from build123d import *

# Parameters (mm, degrees)
SKETCH_1_W      = 3
SKETCH_1_H      = 8
SKETCH_1_W_2    = 8
SKETCH_1_H_2    = 3
EXTRUDE_1_DEPTH = 5


with BuildPart() as part:
    # Эскиз1 → Бобышка-Вытянуть1 (new body)
    with BuildSketch(Plane.XY):
        with BuildLine():
            Line((-31.75, 40.340066927), (-42.5, 40.340066927))
            ThreePointArc((-42.5, 40.340066927), (-43.914213562, 39.754280489), (-44.5, 38.340066927))
            Line((-44.5, 38.340066927), (-44.5, 27.590066927))
            Line((-44.5, 27.590066927), (-42, 27.590066927))
            Line((-42, 27.590066927), (-42, 30.090066927))
            Line((-42, 30.090066927), (-39.5, 30.090066927))
            Line((-39.5, 30.090066927), (-39.5, 21.590066927))
            Line((-39.5, 21.590066927), (-42, 21.590066927))
            Line((-42, 21.590066927), (-42, 24.090066927))
            Line((-42, 24.090066927), (-44.5, 24.090066927))
            Line((-44.5, 24.090066927), (-44.5, -32.409933073))
            Line((-44.5, -32.409933073), (-42, -32.409933073))
            Line((-42, -32.409933073), (-42, -29.909933073))
            Line((-42, -29.909933073), (-39.5, -29.909933073))
            Line((-39.5, -29.909933073), (-39.5, -38.409933073))
            Line((-39.5, -38.409933073), (-42, -38.409933073))
            Line((-42, -38.409933073), (-42, -35.909933073))
            Line((-42, -35.909933073), (-44.5, -35.909933073))
            Line((-44.5, -35.909933073), (-44.5, -46.659933073))
            ThreePointArc((-44.5, -46.659933073), (-43.914213562, -48.074146635), (-42.5, -48.659933073))
            Line((-42.5, -48.659933073), (-31.75, -48.659933073))
            Line((-31.75, -48.659933073), (-31.75, -46.159933073))
            Line((-31.75, -46.159933073), (-34.25, -46.159933073))
            Line((-34.25, -46.159933073), (-34.25, -43.659933073))
            Line((-34.25, -43.659933073), (-25.75, -43.659933073))
            Line((-25.75, -43.659933073), (-25.75, -46.159933073))
            Line((-25.75, -46.159933073), (-28.25, -46.159933073))
            Line((-28.25, -46.159933073), (-28.25, -48.659933073))
            Line((-28.25, -48.659933073), (28.25, -48.659933073))
            Line((28.25, -48.659933073), (28.25, -46.159933073))
            Line((28.25, -46.159933073), (25.75, -46.159933073))
            Line((25.75, -46.159933073), (25.75, -43.659933073))
            Line((25.75, -43.659933073), (34.25, -43.659933073))
            Line((34.25, -43.659933073), (34.25, -46.159933073))
            Line((34.25, -46.159933073), (31.75, -46.159933073))
            Line((31.75, -46.159933073), (31.75, -48.659933073))
            Line((31.75, -48.659933073), (42.5, -48.659933073))
            ThreePointArc((42.5, -48.659933073), (43.914213562, -48.074146635), (44.5, -46.659933073))
            Line((44.5, -46.659933073), (44.5, -35.909933073))
            Line((44.5, -35.909933073), (42, -35.909933073))
            Line((42, -35.909933073), (42, -38.409933073))
            Line((42, -38.409933073), (39.5, -38.409933073))
            Line((39.5, -38.409933073), (39.5, -29.909933073))
            Line((39.5, -29.909933073), (42, -29.909933073))
            Line((42, -29.909933073), (42, -32.409933073))
            Line((42, -32.409933073), (44.5, -32.409933073))
            Line((44.5, -32.409933073), (44.5, 24.090066927))
            Line((44.5, 24.090066927), (42, 24.090066927))
            Line((42, 24.090066927), (42, 21.590066927))
            Line((42, 21.590066927), (39.5, 21.590066927))
            Line((39.5, 21.590066927), (39.5, 30.090066927))
            Line((39.5, 30.090066927), (42, 30.090066927))
            Line((42, 30.090066927), (42, 27.590066927))
            Line((42, 27.590066927), (44.5, 27.590066927))
            Line((44.5, 27.590066927), (44.5, 38.340066927))
            ThreePointArc((44.5, 38.340066927), (43.914213562, 39.754280489), (42.5, 40.340066927))
            Line((42.5, 40.340066927), (31.75, 40.340066927))
            Line((31.75, 40.340066927), (31.75, 37.840066927))
            Line((31.75, 37.840066927), (34.25, 37.840066927))
            Line((34.25, 37.840066927), (34.25, 35.340066927))
            Line((34.25, 35.340066927), (25.75, 35.340066927))
            Line((25.75, 35.340066927), (25.75, 37.840066927))
            Line((25.75, 37.840066927), (28.25, 37.840066927))
            Line((28.25, 37.840066927), (28.25, 40.340066927))
            Line((28.25, 40.340066927), (-28.25, 40.340066927))
            Line((-28.25, 40.340066927), (-28.25, 37.840066927))
            Line((-28.25, 37.840066927), (-25.75, 37.840066927))
            Line((-25.75, 37.840066927), (-25.75, 35.340066927))
            Line((-25.75, 35.340066927), (-34.25, 35.340066927))
            Line((-34.25, 35.340066927), (-34.25, 37.840066927))
            Line((-34.25, 37.840066927), (-31.75, 37.840066927))
            Line((-31.75, 37.840066927), (-31.75, 40.340066927))
        make_face()
        with Locations((-33, 12.5)):
            Rectangle(SKETCH_1_W, SKETCH_1_H, mode=Mode.SUBTRACT)
        with Locations((-32.461916363, -12.5)):
            Rectangle(SKETCH_1_W, SKETCH_1_H, mode=Mode.SUBTRACT)
        with Locations((-16, 12.5)):
            Rectangle(SKETCH_1_W, SKETCH_1_H, mode=Mode.SUBTRACT)
        with Locations((-15.461916363, -12.5)):
            Rectangle(SKETCH_1_W, SKETCH_1_H, mode=Mode.SUBTRACT)
        with Locations((15.5, 13.340066927)):
            Rectangle(SKETCH_1_W_2, SKETCH_1_H_2, mode=Mode.SUBTRACT)
        with Locations((15.5, 30.340066927)):
            Rectangle(SKETCH_1_W_2, SKETCH_1_H_2, mode=Mode.SUBTRACT)
        with Locations((15.5, -12.659933073)):
            Rectangle(SKETCH_1_W_2, SKETCH_1_H_2, mode=Mode.SUBTRACT)
        with Locations((15.5, 4.340066927)):
            Rectangle(SKETCH_1_W_2, SKETCH_1_H_2, mode=Mode.SUBTRACT)
        with Locations((15.5, -38.659933073)):
            Rectangle(SKETCH_1_W_2, SKETCH_1_H_2, mode=Mode.SUBTRACT)
        with Locations((15.5, -21.659933073)):
            Rectangle(SKETCH_1_W_2, SKETCH_1_H_2, mode=Mode.SUBTRACT)
    extrude(amount=EXTRUDE_1_DEPTH)


solid = part.part
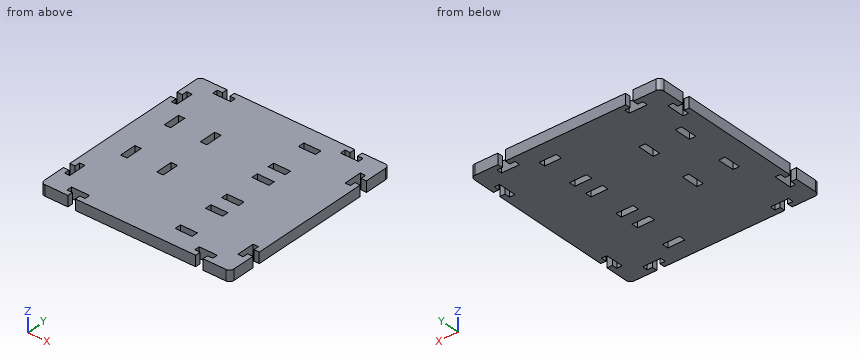
Geometry check sheet. Reference: the model listing, model coordinates, mm. Give positions to 0.01 mm unless a question says otherwise; leave off trailing zeros. Loops run counter-clockwise (first coordinate to the right, second up) from the corner with the lowest first, then second, coordinate; pieces in that order, holes last. Notation, with made-up numbers: (65.25, 9.5) -> (73.25, 9.5) arc R13 ccw to (73.25, 20.5) -> close; hole circle Ø1 at (-18, -25). An arc over 180 degrees is marked (long way). Answer in a Markdown table with one row per item. Add a question column.
1) Cross-section at A-A on y = -10. Record the boundary of the cut face in (x, z), and give its area (3 significant figures).
2) Gauge pin test, flat ends, axial feed: P1, Ø2, axis at y = 38.5, z = 3, coming from the -X side; P2, Ø1.2, axis at x = 43.5, z = 2, coming from the +Y side. Record the tip position at first contact, or that the pin passes through.
3) Cross-section at B-B on x = 17. Record the boundary of the cut face in (y, z).
4) Cross-section at C-C on z = 2.5. State how many separate pieces and enclosed holes the cut face has, and give its area (3 significant figures).
5) Material ranges on probe 1 along Y at (x, z) = (-27, 2.2); probe 2 along Y at (x, z) = (41, 0.8); probe 3 along X at (y, z) = (23.5, 0.3), recorded low to high. Write a range as from..to.
Outcome:
| question | item | result |
|---|---|---|
| 1 | outline | (-44.5, 0) -> (-33.96, 0) -> (-33.96, 5) -> (-44.5, 5) -> close; (-30.96, 0) -> (-16.96, 0) -> (-16.96, 5) -> (-30.96, 5) -> close; (-13.96, 0) -> (44.5, 0) -> (44.5, 5) -> (-13.96, 5) -> close |
| 1 | area | 415 mm^2 |
| 2 | P1 | stops at x = -44.5 |
| 2 | P2 | stops at y = 40.3 |
| 3 | outline | (-48.66, 0) -> (-40.16, 0) -> (-40.16, 5) -> (-48.66, 5) -> close; (-37.16, 0) -> (-23.16, 0) -> (-23.16, 5) -> (-37.16, 5) -> close; (-20.16, 0) -> (-14.16, 0) -> (-14.16, 5) -> (-20.16, 5) -> close; (-11.16, 0) -> (2.84, 0) -> (2.84, 5) -> (-11.16, 5) -> close; (5.84, 0) -> (11.84, 0) -> (11.84, 5) -> (5.84, 5) -> close; (14.84, 0) -> (28.84, 0) -> (28.84, 5) -> (14.84, 5) -> close; (31.84, 0) -> (40.34, 0) -> (40.34, 5) -> (31.84, 5) -> close |
| 4 | separate pieces | 1 |
| 4 | enclosed holes | 10 |
| 4 | area | 7,440 mm^2 |
| 5 | probe 1 | y = -48.66..-46.16, -43.66..35.34, 37.84..40.34 |
| 5 | probe 2 | y = -48.66..-38.41, -29.91..21.59, 30.09..40.34 |
| 5 | probe 3 | x = -44.5..-42, -39.5..39.5, 42..44.5 |
